Input: dimensioned drawing with shaded views. Units: mm. Origin: part minimum x, y, z. Round coordinates to 2 decimals unless told otherwise and drop trailing zeros. Loops run counter-clockwise (first coordinate to the right, second up) from the corner with the lowest first, then second, coordinate; pieces in that order, holes last. Notation, with made-up numbers: (-22.75, -10) - (-13.75, -10) arc R19 ccw to (-13.75, 7) - close; hole circle Ø8 at (65.25, 86.25). An arc over 180 degrees is marked (long way). One line per question, with ' | ' between items.
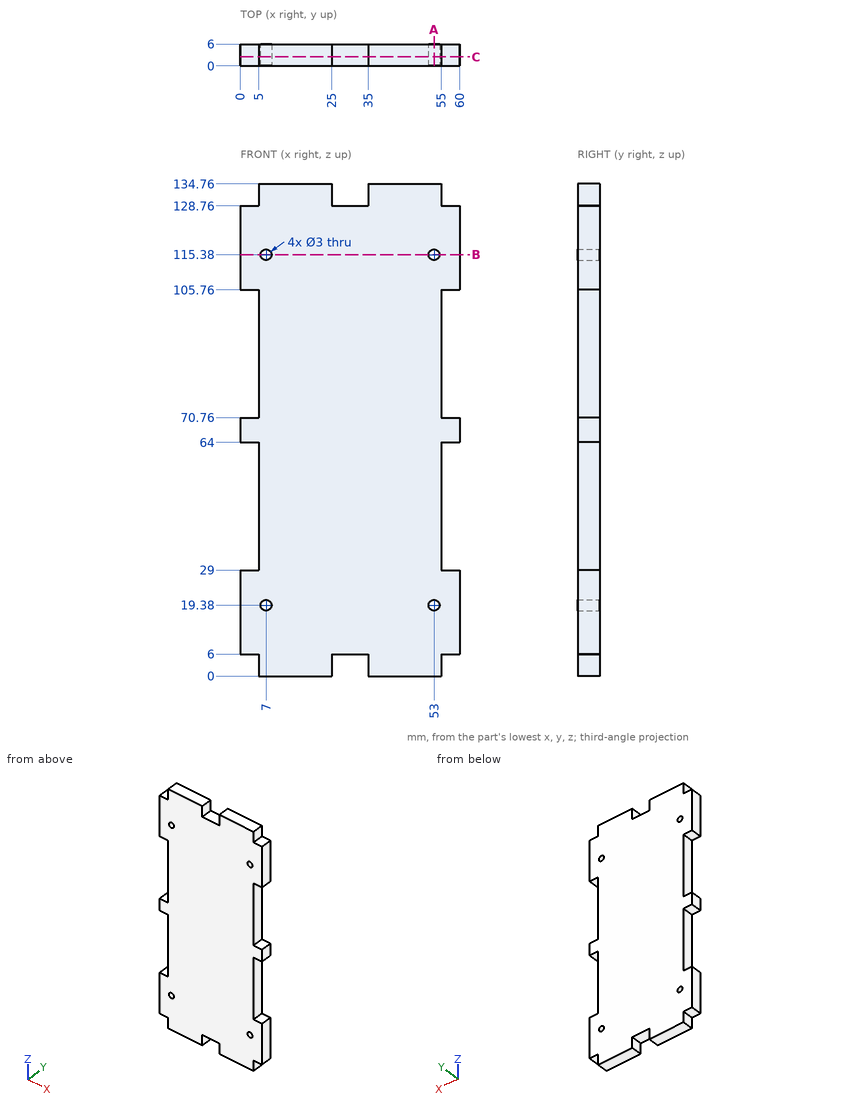
1. Section query A-A, the plane x = 53. Return loops of the section in (y, z), plus the area to 3 significant figures.
Worked out:
outline: (0, 0) - (6, 0) - (6, 17.88) - (0, 17.88) - close; (0, 20.88) - (6, 20.88) - (6, 113.88) - (0, 113.88) - close; (0, 116.88) - (6, 116.88) - (6, 134.76) - (0, 134.76) - close | area: 773 mm2
2. Section query B-B, the plane z = 115.38. Return loops of the section in (x, y), plus the area to 3 significant figures.
Worked out:
outline: (0, 0) - (5.5, 0) - (5.5, 6) - (0, 6) - close; (8.5, 0) - (51.5, 0) - (51.5, 6) - (8.5, 6) - close; (54.5, 0) - (60, 0) - (60, 6) - (54.5, 6) - close | area: 324 mm2
3. Material intervals for probe 1 along Z at (x, y) = (53, 3.65); probe 2 along Z at (x, y) = (4, 2.4); probe 3 along X at (y, z) = (3.1, 115.38), sorted ascending.
Worked out:
probe 1: z = 0 to 17.88, 20.88 to 113.88, 116.88 to 134.76 | probe 2: z = 6 to 29, 64 to 70.76, 105.76 to 128.76 | probe 3: x = 0 to 5.5, 8.5 to 51.5, 54.5 to 60
4. Contact query for flat-ended pins moving along their axis: P1, Ø3, axis at y = 1.5, z = 132, coming from the +X side; P2, Ø1.5, axis at x = 1.5, y = 2.5, coming from the +Z side; P3, Ø1, axis at y = 4, z = 46, coming from the -X side; P4, Ø1.8, axis at x = 53, z = 19.38, coming from the -Y side. Output: stop coordinate, or through.
Worked out:
P1: stops at x = 55 | P2: stops at z = 128.76 | P3: stops at x = 5 | P4: passes through
5. Section query C-C, the plane y = 2.5. Give the number of separate pieces and of enclosed holes in the cut face, plus the area to 3 significant figures.
Worked out:
separate pieces: 1 | enclosed holes: 4 | area: 7,120 mm2
